Print and shaded views of the part. All mm, measured from the part's lowest x, y and z. A direction names the side the tool comes from. Coordinates: 2 decimals unless noted, no trailing zeros. Order: outer loops, then holes, each group sorted by start corner. A loop starts at its lowest first (then second) coordinate and runs counter-clockwise, first axis right, second up. Notation, with made-up numbers: M 8,24 L 16,24 A26 ccw 16,47 Z; hole C -36.75,13 d10. An arc over 180 degrees is marked long. One line per item, written item: value.
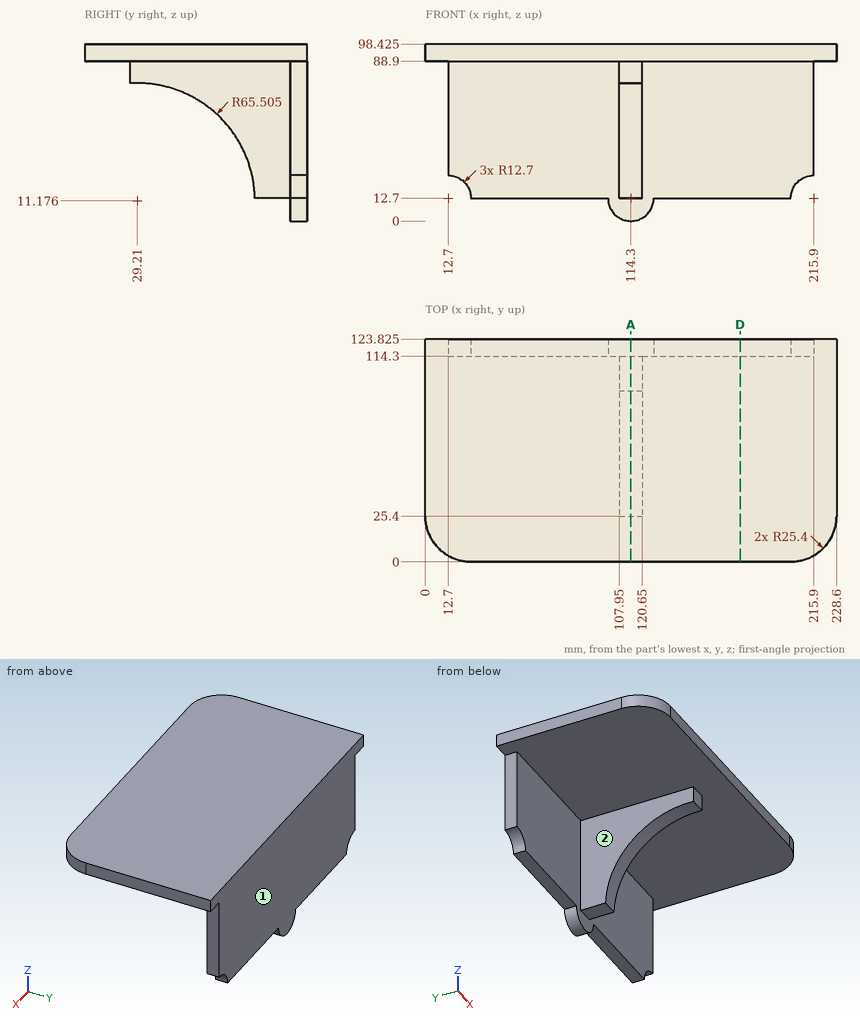
Q1. Pin check, flat tips, straight feed: pin 1 Ø5 at (y, z) = (117, 48) entering from -X; pin 2 Ø7.5 at (x, y) = (58, 118) entering from -Z; pin 3 Ø6 at (x, z) = (114, 84.5) entering from -Y. Stop position of each tip, or through.
Recorded:
pin 1: stops at x = 12.7
pin 2: stops at z = 12.7
pin 3: stops at y = 25.4
Q2. Which spindle directions (+Z, -Z, +X, -X, +Y, -Y) get a long thin tool onto all of the face, cutting with end or side? Do the marked faces 1 and 2. Say none if no direction does.
Recorded:
face 1: +Z, -Z, +X, -X, +Y
face 2: -Z, -X, -Y
Q3. Drill centre lines: line 1 along Y through (x, z) = (128, 69.5) (1 decimal); line 2 along Z through (x, y) = (209, 91) (1 decimal); line 3 along X through (y, z) = (106, 63.5). Where is each one in solid material? Low to high.
Recorded:
line 1: y = 114.3 to 123.8
line 2: z = 88.9 to 98.4
line 3: x = 107.95 to 120.65
Q4. Slice it at D-D (x = 175). List the corners of the cut face in (y, z) (1 decimal).
Recorded:
outline: M 0,88.9 L 114.3,88.9 L 114.3,12.7 L 123.8,12.7 L 123.8,98.4 L 0,98.4 Z
Q5. Slice it at A-A (x = 114.3). List the corners of the cut face in (y, z) (1 decimal).
Recorded:
outline: M 0,88.9 L 25.4,88.9 L 25.4,76.6 A65.5 cw 94.7,12.7 L 114.3,12.7 L 114.3,0 L 123.8,0 L 123.8,98.4 L 0,98.4 Z
